Input: part model. Units: mm. Frame: model coordinates. Face numbers are marked on the shaded views. A direction names the side the tool comes from. Coordinates: 2 decimals unless noted, no trailing zeros. Order: outer loops, then holes, each group sorted by start corner. A loop starts at its lowest first (then second) coordinate and runs counter-clockwise, first axis right, second up. Notation, with made-up numbers: M -38,-39.5 L 18,-39.5 A33 cw 18,-8.5 Z; hole C -29,-37.5 d3. An arc over 180 degrees is marked long. Answer in a Markdown table with one row per item.
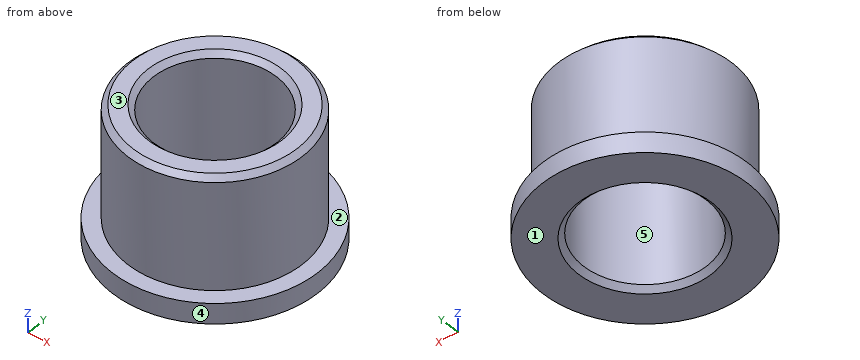
from build123d import *

# Parameters (mm, degrees)
SKETCH_1_R          = 10
EXTRUDE_1_DEPTH     = 2
SKETCH_2_R          = 8.5
EXTRUDE_2_DEPTH     = 13
SKETCH_3_R          = 6
CUT_EXTRUDE_1_DEPTH = 20.209372712
CHAMFER_1_SIZE      = 0.5


with BuildPart() as part:
    # 草图1 → 凸台-拉伸1 (new body)
    with BuildSketch(Plane.XY):
        Circle(SKETCH_1_R)
    extrude(amount=EXTRUDE_1_DEPTH)

    # 草图2 → 凸台-拉伸2 (add)
    with BuildSketch(Plane.XY):
        with Locations(Location((0, 0, 0), (0, 0, 180))):
            Circle(SKETCH_2_R)
    extrude(amount=EXTRUDE_2_DEPTH)

    # 草图3 → 切除-拉伸1 (cut, through all)
    with BuildSketch(Plane.XY.offset(13)):
        Circle(SKETCH_3_R)
    extrude(amount=-CUT_EXTRUDE_1_DEPTH, mode=Mode.SUBTRACT)

    # 倒角1
    chamfer_1_edges = [part.edges().sort_by_distance(p)[0] for p in [
        (-6, 0, 0),
        (-6, 0, 13),
        (8.5, 0, 13),
    ]]
    chamfer(chamfer_1_edges, length=CHAMFER_1_SIZE)


solid = part.part
1) Material intervals for probe 1 along Y at (x, z) = (0, 3.75); probe 2 along X at (y, z) = (0.25, 6.75); probe 3 along Z at (x, y) = (2.75, 8.5), sorted ascending.
Resolved:
| item | result |
|---|---|
| probe 1 | y = -8.5 to -6, 6 to 8.5 |
| probe 2 | x = -8.5 to -5.99, 5.99 to 8.5 |
| probe 3 | z = 0 to 2 |
2) Mould query, pull axis Y, two halves, no side actions, for the marked faces 3, 4 and 5. Classes: +Y half, -Y half, draft (parallel to the pull), parting line (faces both ways), or undercut.
Resolved:
| item | result |
|---|---|
| face 3 | draft |
| face 4 | parting line |
| face 5 | undercut |
3) Reachability of the marked faces 1 and 2 from +Z, -Z, +X, -X, +Y, -Y: full face, straight path, thin tool, end or side. Return the list, or none.
Resolved:
| item | result |
|---|---|
| face 1 | -Z, +X, -X, +Y, -Y |
| face 2 | +Z |
4) Cut plane D-D, the plane y = -9. Output: boundary loops of the cut face in (x, z).
Resolved:
| item | result |
|---|---|
| outline | M -4.36,0 L 4.36,0 L 4.36,2 L -4.36,2 Z |
5) Cut plane C-C, the plane z = 10.5. Output: boundary loops of the cut face in (x, y).
Resolved:
| item | result |
|---|---|
| outline | C 0,0 d17; hole C 0,0 d12 |
6) Contact query for flat-ended pins moving along their axis: pin 1 (5 mm diameter, centred on x = -0.5, z = 9, fed in from +Y); pin 2 (10 mm diameter, centred on x = 1, y = -1, fed in from +Z); pin 3 (1.5 mm diameter, centred on y = 2.5, z = 4.5, fed in from -X). Output: stop coordinate, or through.
Resolved:
| item | result |
|---|---|
| pin 1 | stops at y = 8.5 |
| pin 2 | stops at z = 12.91 |
| pin 3 | stops at x = -8.32 |
7) Cut plane A-A, the plane y = 0. Output: boundary loops of the cut face in (x, z).
Resolved:
| item | result |
|---|---|
| outline | M -10,0 L -6.5,0 L -6,0.5 L -6,12.5 L -6.5,13 L -8,13 L -8.5,12.5 L -8.5,2 L -10,2 Z; M 6,0.5 L 6.5,0 L 10,0 L 10,2 L 8.5,2 L 8.5,12.5 L 8,13 L 6.5,13 L 6,12.5 Z |
